The figure shows three views and two pictorial views of one solid part (mm, origin at its lowest corner). Answer the questions. A direction names the side the tool comes from. Give positions to 0.01 mm unless a question says otherwise; leave off trailing zeros. Write each loop counter-clockwise with the first axis right and the second up, starting at its lowest first coordinate (ties: lowest second). Pieces come first, ordered by that corner, then holes. Notation, with made-up numbers: (-18, 46) -> (37, 46) arc R10 cw to (37, 50) -> close; hole circle Ø6 at (18, -19). An arc over 180 degrees is marked (long way). Write item = value, one per line. Start each with the question number.
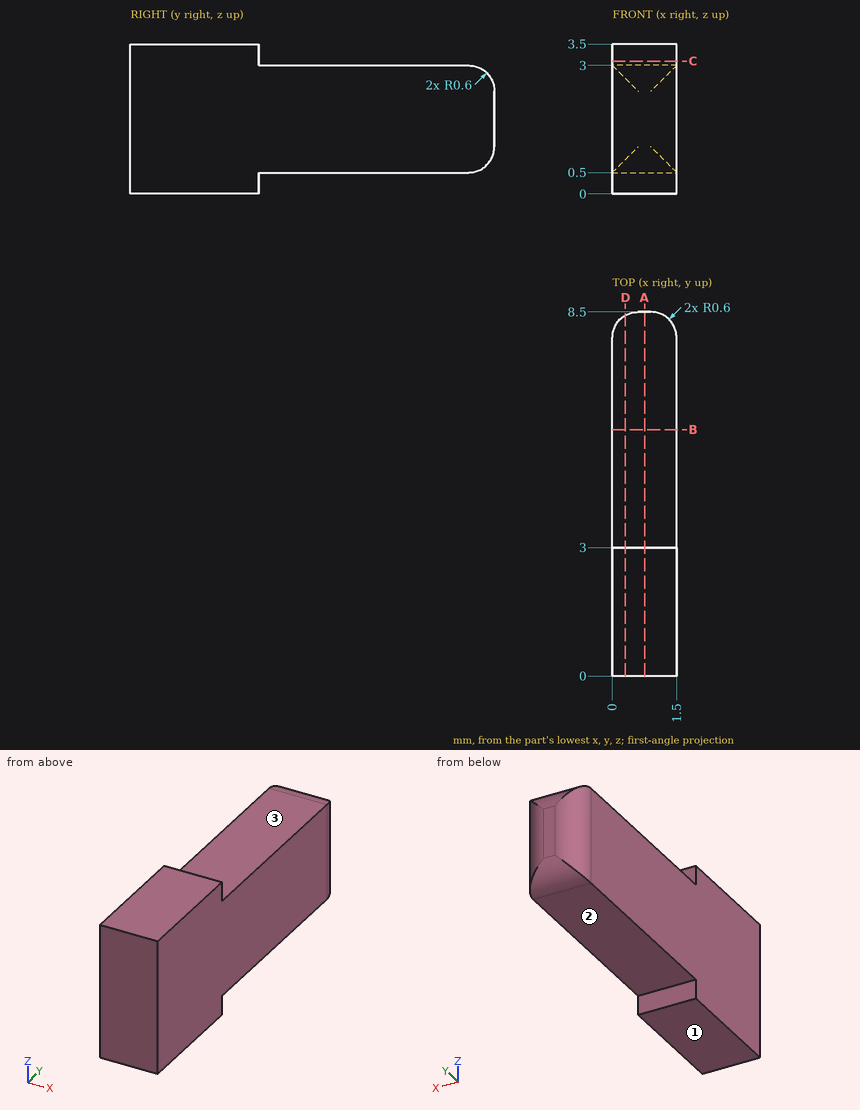
(1) A cutting plane is placed at B-B, the plane y = 5.75. Write down the section's boundary in (x, z), then the cut area to 3 significant figures.
(2) A cutting plane is placed at C-C, the plane z = 3.1. Write down the section's boundary in (x, y), then the cut area to 3 significant figures.
(3) A cutting plane is placed at D-D, the plane x = 0.3. Write down the section's boundary in (y, z).
(4) Find the intervals of material crossed by line 1 along Z through (x, y) = (0.4, 6); line 2 along Y through (x, z) = (0.2, 3.35); line 3 along Y through (x, z) = (1, 2.2), in increasing order.
(5) A cutting plane is placed at A-A, the plane x = 0.75. Write down the section's boundary in (y, z), then the cut area to 3 significant figures.
(6) For the marked faces 1, 2 and 3, determine the directions among +Z, -Z, +X, -X, +Y, -Y from which every point of the face is accessible in a straight line to the end or side of a thin tool.
Results list:
q1.outline = (0, 0.5) -> (1.5, 0.5) -> (1.5, 3) -> (0, 3) -> close
q1.area = 3.75 mm²
q2.outline = (0, 0) -> (1.5, 0) -> (1.5, 3) -> (0, 3) -> close
q2.area = 4.50 mm²
q3.outline = (0, 0) -> (3, 0) -> (3, 0.5) -> (7.9, 0.5) arc R0.6 ccw to (8.42, 0.8) -> (8.42, 2.7) arc R0.6 ccw to (7.9, 3) -> (3, 3) -> (3, 3.5) -> (0, 3.5) -> close
q4.line_1 = 0.5 to 3
q4.line_2 = 0 to 3
q4.line_3 = 0 to 8.49
q5.outline = (0, 0) -> (3, 0) -> (3, 0.5) -> (7.9, 0.5) arc R0.6 ccw to (8.5, 1.1) -> (8.5, 2.4) arc R0.6 ccw to (7.9, 3) -> (3, 3) -> (3, 3.5) -> (0, 3.5) -> close
q5.area = 24.1 mm²
q6.face_1 = -Z, +X, -X, +Y, -Y
q6.face_2 = -Z, +X, -X, +Y
q6.face_3 = +Z, +X, -X, +Y
